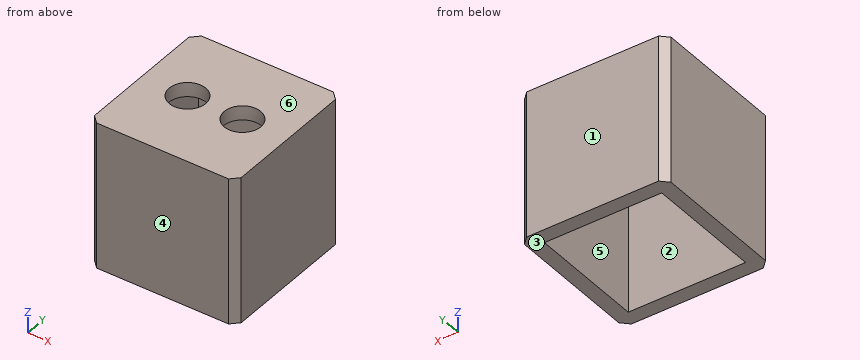
```python
from build123d import *

# Parameters (mm, degrees)
ESQUISSE1_W                       = 20
ESQUISSE1_H                       = 20
BOSS_EXTRU_1_DEPTH                = 20
ENL_V_START                       = -3
ESQUISSE2_R                       = 2.6
ENL_V_MAT_EXTRU_1_DEPTH           = 53.506491459
ENL_V_MAT_EXTRU_1_DRAFT           = 2
ENL_V_MAT_EXTRU_1_PROFILE_2_DEPTH = 53.506491459
ENL_V_MAT_EXTRU_1_PROFILE_2_DRAFT = 2
ESQUISSE3_W                       = 16
ESQUISSE3_H                       = 16
ENL_V_MAT_EXTRU_2_DEPTH           = 18
CHANFREIN1_SIZE                   = 1


with BuildPart() as part:
    # Esquisse1 → Boss.-Extru.1 (new body)
    with BuildSketch(Plane.XY):
        with Locations((-24.630410255, 19.182655502)):
            Rectangle(ESQUISSE1_W, ESQUISSE1_H)
    extrude(amount=BOSS_EXTRU_1_DEPTH)


with BuildPart() as enl_v_mat_extru_1_tool:
    # Esquisse2 → Enlèv. mat.-Extru.1 (with draft: the straight prism first)
    with BuildSketch(Plane.XY.offset(20).offset(ENL_V_START)):
        with Locations((-28.380410255, 19.182655502)):
            Circle(ESQUISSE2_R)
    extrude(amount=ENL_V_MAT_EXTRU_1_DEPTH)
    # Enlèv. mat.-Extru.1: the draft: its side faces are tilted about the plane it starts from
    enl_v_mat_extru_1_sides = [enl_v_mat_extru_1_tool.faces().sort_by_distance(p)[0] for p in [
        (-30.980410255, 19.182655502, 43.75324573),
    ]]
    draft(enl_v_mat_extru_1_sides, Plane.XY.offset(20).offset(ENL_V_START), ENL_V_MAT_EXTRU_1_DRAFT)


with BuildPart() as part_1:
    add(part.part)

    # Enlèv. mat.-Extru.1: cut by enl_v_mat_extru_1_tool
    add(enl_v_mat_extru_1_tool.part, mode=Mode.SUBTRACT)


with BuildPart() as enl_v_mat_extru_1_profile_2_tool:
    # Esquisse2 → Enlèv. mat.-Extru.1 profile 2 (with draft: the straight prism first)
    with BuildSketch(Plane.XY.offset(20).offset(ENL_V_START)):
        with Locations((-20.880410255, 19.182655502)):
            Circle(ESQUISSE2_R)
    extrude(amount=ENL_V_MAT_EXTRU_1_PROFILE_2_DEPTH)
    # Enlèv. mat.-Extru.1 profile 2: the draft: its side faces are tilted about the plane it starts from
    enl_v_mat_extru_1_profile_2_sides = [enl_v_mat_extru_1_profile_2_tool.faces().sort_by_distance(p)[0] for p in [
        (-23.480410255, 19.182655502, 43.75324573),
    ]]
    draft(enl_v_mat_extru_1_profile_2_sides, Plane.XY.offset(20).offset(ENL_V_START), ENL_V_MAT_EXTRU_1_PROFILE_2_DRAFT)


with BuildPart() as part_2:
    add(part_1.part)

    # Enlèv. mat.-Extru.1 profile 2: cut by enl_v_mat_extru_1_profile_2_tool
    add(enl_v_mat_extru_1_profile_2_tool.part, mode=Mode.SUBTRACT)

    # Esquisse3 → Enlèv. mat.-Extru.2 (cut)
    with BuildSketch(Plane(origin=(0, 0, 0), x_dir=(-1, 0, 0), z_dir=(0, 0, -1))):
        with Locations((24.630410255, 19.182655502)):
            Rectangle(ESQUISSE3_W, ESQUISSE3_H)
    extrude(amount=-ENL_V_MAT_EXTRU_2_DEPTH, mode=Mode.SUBTRACT)

    # Chanfrein1
    chanfrein1_edges = [part_2.edges().sort_by_distance(p)[0] for p in [
        (-34.630410255, 29.182655502, 10),
        (-14.630410255, 29.182655502, 10),
        (-14.630410255, 9.182655502, 10),
        (-34.630410255, 9.182655502, 10),
    ]]
    chamfer(chanfrein1_edges, length=CHANFREIN1_SIZE)


solid = part_2.part
```
Could you check a few things on this model? Use its own coordinates, in mm. Face numbers are marked on the shaded views. A direction names the side the tool comes from. Give positions to 0.01 mm unless a question says otherwise; leave off trailing zeros. Order: outer loops, then holes, each group sorted by start corner. A loop starts at its lowest first (then second) coordinate and runs counter-clockwise, first axis right, second up.
Q1. If I drill on line 1 along Y through (x, z) = (-26.75, 7.5); line 2 along X through (y, z) = (18.25, 14); line 3 along X through (y, z) = (19.5, 18.5), over which ranges is the centre line in solid material (lowest first)?
Q2. Suppose I cut it at A-A, the plane z = 9.25. Write out the boundary of the cut face in (x, y), and give its area (3 significant figures).
Q3. I'm going to push a flat-ended pin straight in: P1, Ø1.5, axis at x = -18.5, y = 22, coming from the -Z side. Where does the tip first touch, or does it pass through?
Q4. Suppose I cut it at C-C, the plane x = -17. Write out the boundary of the cut face in (y, z).
Q5. For the marked faces 5 and 6, which set-ups out of +Z, -Z, +X, -X, +Y, -Y let a thin tool reach every point of the face, with its end or its side?
Q6. Suppose I cut it at B-B, the plane y = 25.75. Write out the boundary of the cut face in (x, z), and give its area (3 significant figures).
Q7. We'd pull the mould along Y, two halves only. Please class the marked faces 1, 2, 3 and 4: +Y half, -Y half, draft (parallel to the pull), parting line (faces both ways), or undercut.
Q8. Suppose I cut it at D-D, the plane y = 19.5. Count the separate pieces of the cut face and the enclosed holes in it, and give its area (3 significant figures).
Solution:
1. line 1: y = 9.18 to 11.18, 27.18 to 29.18
1. line 2: x = -34.63 to -32.63, -16.63 to -14.63
1. line 3: x = -34.63 to -30.91, -25.85 to -23.41, -18.35 to -14.63
2. outline: (-34.63, 10.18) - (-33.63, 9.18) - (-15.63, 9.18) - (-14.63, 10.18) - (-14.63, 28.18) - (-15.63, 29.18) - (-33.63, 29.18) - (-34.63, 28.18) - close; hole (-32.63, 11.18) - (-16.63, 11.18) - (-16.63, 27.18) - (-32.63, 27.18) - close
2. area: 142 mm2
3. P1: stops at z = 18
4. outline: (9.18, 0) - (11.18, 0) - (11.18, 18) - (27.18, 18) - (27.18, 0) - (29.18, 0) - (29.18, 20) - (9.18, 20) - close
5. face 5: -Z
5. face 6: +Z, +X, -X, +Y, -Y
6. outline: (-34.63, 0) - (-32.63, 0) - (-32.63, 18) - (-16.63, 18) - (-16.63, 0) - (-14.63, 0) - (-14.63, 20) - (-34.63, 20) - close
6. area: 112 mm2
7. face 1: +Y half
7. face 2: undercut
7. face 3: draft
7. face 4: -Y half
8. separate pieces: 3
8. enclosed holes: 0
8. area: 91.9 mm2
